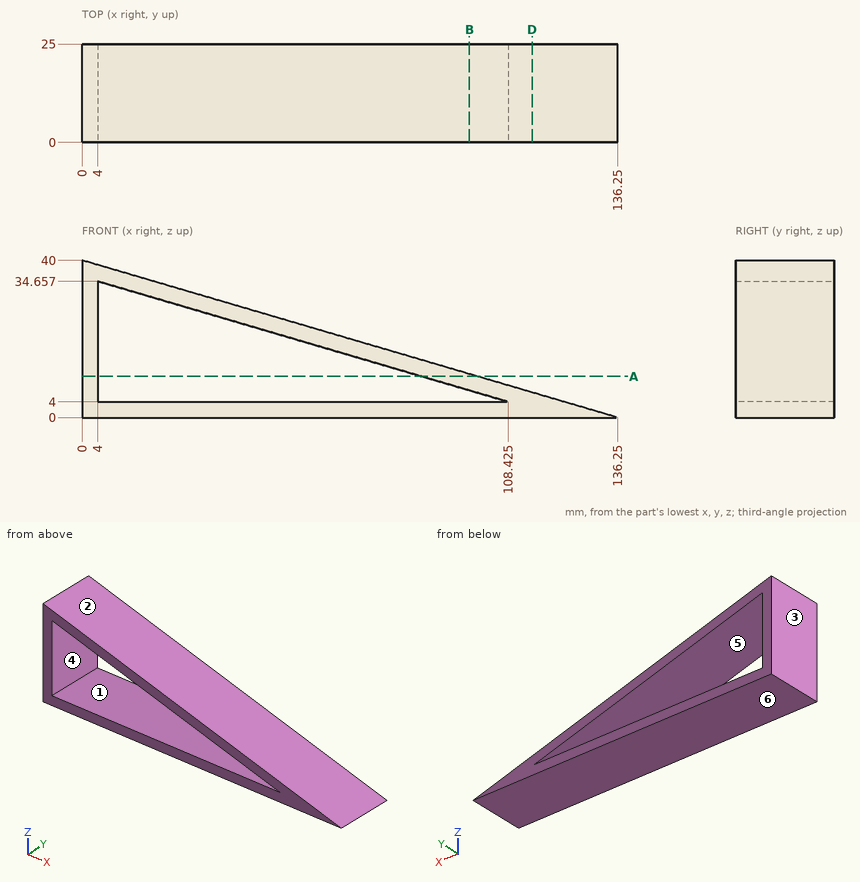
Input: dimensioned drawing with shaded views. Units: mm. Origin: part minimum x, y, z. A direction names the side the tool comes from. Round coordinates to 2 decimals unless told otherwise and drop trailing zeros. Order: outer loops, then holes, each group sorted by start corner. A loop starts at its lowest first (then second) coordinate and runs counter-clockwise, first axis right, second up. Notation, with made-up numbers: (-31.75, -24.5) - (-17.75, -24.5) arc R25 ccw to (-17.75, 3.5) - close; hole circle Ø2 at (-27, -16). An arc over 180 degrees is marked (long way). Write item = value, one per line. Start each with the question number.
Q1. Pin query (flat end, axial travel): pin 1 (2 mm diameter, centred on x = 48, y = 6.5, fed in from +Z); pin 2 (10 mm diameter, centred on x = 48.5, y = 20.5, fed in from +Z). Return the tip coordinate at first contact, or that it passes through.
Q2. Cut plane D-D on x = 114.5. Return the cut outline in (y, z) (1 decimal), and give its area (3 significant figures).
Q3. Cut plane A-A on z = 10.5. Return the cut outline in (x, y).
Q4. Access query for the marked faces 1 and 2. Directions: +Z, -Z, +X, -X, +Y, -Y. A direction counts if a zero-diameter tool reaches every point of the face in a straight line with its end or side. Return the directions, or none.
Q5. Pull-direction query (Z, two-part tool) for the marked faces 3, 4, 5 and 6; classes: +Z half, -Z half, draft (parallel to the pull), parting line (faces both ways), or undercut.
Q6. Ray query, line 1 (Z direction, x = 69, y = 2.25) (1 decimal); line 2 (Z direction, x = 21, y = 17.25) (1 decimal); line 3 (Z direction, x = 126, y = 3). Return the intervals inside material, ascending. Write a range as from..to.
Q7. Cut plane B-B on x = 98.5. Return the cut outline in (y, z).
Outcome:
q1.pin_1 = 26.2
q1.pin_2 = 27.23
q2.outline = (0, 0) - (25, 0) - (25, 6.4) - (0, 6.4) - close
q2.area = 160 mm^2
q3.outline = (0, 0) - (4, 0) - (4, 25) - (0, 25) - close; (86.28, 0) - (100.48, 0) - (100.48, 25) - (86.28, 25) - close
q4.face_1 = +Y, -Y
q4.face_2 = +Z, +X, +Y, -Y
q5.face_3 = draft
q5.face_4 = undercut
q5.face_5 = undercut
q5.face_6 = -Z half
q6.line_1 = 0..4, 15.6..19.7
q6.line_2 = 0..4, 29.7..33.8
q6.line_3 = 0..3.01
q7.outline = (0, 0) - (25, 0) - (25, 4) - (0, 4) - close; (0, 6.91) - (25, 6.91) - (25, 11.08) - (0, 11.08) - close
